Build history of the part. All positions in model axes, mm. Face numbers are marked on the shaded views. A direction names the side the tool comes from. Round coordinates to 2 decimals unless told otherwise and drop trailing zeros. Loops run counter-clockwise (first coordinate to the right, second up) from the corner with the lowest first, then second, coordinate; pieces in that order, holes last. Notation, with made-up numbers: (75, -38.5) - (99, -38.5) arc R13 cw to (99, -30.5) - close; hole circle Ø1 at (33.5, 43). An arc over 180 degrees is marked (long way). Use one line per item in the form item = value. Start each with the question number.
Q1. 3-axis set-ups, long thin cutter, end or side, ignore diameter. For the marked faces 1 and 2: which of +Z, -Z, +X, -X, +Y, -Y reach the whole face in a straight line?
Q2. Pin check, flat tips, straight feed: pin 1 (1 mm diameter, centred on x = 0, z = 14.5, fed in from +Y); pin 2 (3 mm diameter, centred on x = -1.5, z = 16.5, fed in from -Y); pin 3 (3 mm diameter, centred on y = 1, z = 10, fed in from +X). Stop position of each tip, or through.
Q3. Drill centre lines: line 1 (Z direction, x = -0.9, y = 2.5); line 2 (X direction, y = -0.1, z = 16); line 3 (X direction, y = 0.5, z = 4.75). Where is each one in solid material? Low to high.
Q4. Saw through at A-A (y = 0). Give the cut face in (x, z), then the cut area to 3 significant figures.
Q5. Saw through at D-D (x = 2.6). Give the cut face in (y, z).
Q6. Saw through at C-C (z = 17). Give the cut face in (x, y).
```python
from build123d import *

# Parameters (mm, degrees)
SKETCH1_R      = 1.2192
EXTRUDE1_DEPTH = 19.144
SKETCH2_R      = 2.9845
EXTRUDE2_DEPTH = 0.381
SKETCH3_R      = 2.2479
EXTRUDE3_DEPTH = 1.143
FILLET1_R      = 1.016


with BuildPart() as part:
    # Sketch1 → Extrude1 (new body)
    with BuildSketch(Plane.XY):
        Circle(SKETCH1_R)
    extrude(amount=EXTRUDE1_DEPTH)

    # Sketch2 → Extrude2 (add)
    with BuildSketch(Plane(origin=(0, 0, 0), x_dir=(-1, 0, 0), z_dir=(0, 0, -1))):
        Circle(SKETCH2_R)
    extrude(amount=EXTRUDE2_DEPTH)

    # Sketch3 → Extrude3 (add)
    with BuildSketch(Plane(origin=(0, 0, -0.381), x_dir=(-1, 0, 0), z_dir=(0, 0, -1))):
        Circle(SKETCH3_R)
    extrude(amount=EXTRUDE3_DEPTH)

    # Fillet1
    fillet1_edges = [part.edges().sort_by_distance(p)[0] for p in [
        (2.2479, 0, -1.524),
    ]]
    fillet(fillet1_edges, radius=FILLET1_R)


solid = part.part
```
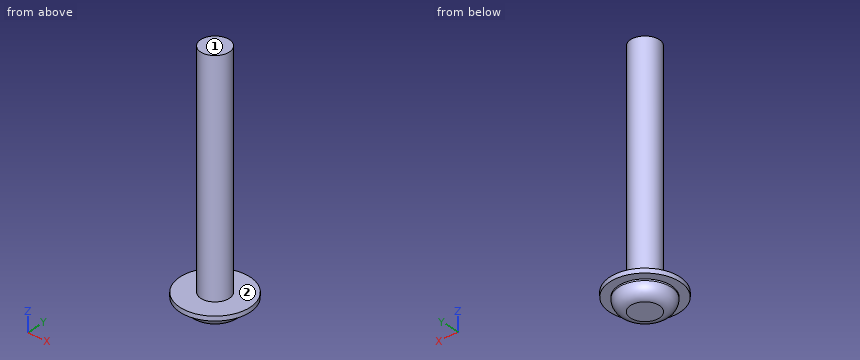
Report:
q1.face_1 = +Z, +X, -X, +Y, -Y
q1.face_2 = +Z
q2.pin_1 = 1.22
q2.pin_2 = -1.22
q2.pin_3 = 1.22
q3.line_1 = -0.38 to 0
q3.line_2 = -1.22 to 1.22
q3.line_3 = -1.11 to 1.11
q4.outline = (-2.98, -0.38) - (-2.25, -0.38) - (-2.25, -0.51) arc R1.02 ccw to (-1.23, -1.52) - (1.23, -1.52) arc R1.02 ccw to (2.25, -0.51) - (2.25, -0.38) - (2.98, -0.38) - (2.98, 0) - (1.22, 0) - (1.22, 19.14) - (-1.22, 19.14) - (-1.22, 0) - (-2.98, 0) - close
q4.area = 53.7 mm²
q5.outline = (-1.47, -0.38) - (1.47, -0.38) - (1.47, 0) - (-1.47, 0) - close
q6.outline = circle Ø2.44 at (0, 0)
